Could you check a few things on this model? Use its own coordinates, in mm. Coordinates: 2 decimals unless noted, no trailing zeros. Write each loop counter-clockwise with the first axis right and the second up, starting at its lowest first coordinate (ties: lowest second). Pieces come first, ordered by that corner, then holes.
Autodesk Inventor part; units mm, degrees
ref_plane "РабПлоскость1" through (0, -6.05, 0) normal (1, 0, 0) x (0, 0, -1)
ref_plane "YZ Plane" through (0, 0, 0) normal (1, 0, 0) x (0, 1, 0)
ref_plane "XZ Plane" through (0, 0, 0) normal (0, 1, 0) x (-1, 0, 0)
sketch "Эскиз1" plane through (0, 0, 0) normal (0, 0, 1) x (1, 0, 0)
  circle A0 centre (0, 0) radius 4.05
  line L0 (-6.05, -6.05) -> (6.05, -6.05)
  line L1 (6.05, -6.05) -> (6.05, 6.05)
  line L2 (6.05, 6.05) -> (-6.05, 6.05)
  line L3 (-6.05, 6.05) -> (-6.05, -6.05)
  line L4 (-6.05, -6.05) -> (6.05, 6.05) construction
  line L5 (6.05, -6.05) -> (-6.05, 6.05) construction
  line L6 (0, 6.05) -> (0, 4.05)
  line L7 (-6.05, 0) -> (-4.05, 0)
  line L8 (-13, -3.05) -> (0, -3.05)
  line L9 (0, -3.05) -> (0, -6.05)
  line L10 (0, -6.05) -> (-13, -6.05)
  line L11 (-13, -6.05) -> (-13, -3.05)
  line L12 (13, -3.05) -> (0, -3.05)
  line L13 (0, -6.05) -> (13, -6.05)
  line L14 (13, -6.05) -> (13, -3.05)
  point P0 (0, -4.55)
  point P1 (0, -6.05)
  point P2 (2.6646, -3.05)
  point P3 (-2.6646, -3.05)
  dimension "d0" = 8.1
  dimension "d1" = 2
  dimension "d2" = 2
  dimension "d3" = 3
  dimension "d5" = 3
  dimension "d6" = 6.95
extrude "Выдавливание1" add sketch "Эскиз1" along normal blind 5.1 contours L12 L1 L0 L9 A0 | L9 L0 L3 L8 A0 | L12 L14 L13 L1 | L3 L10 L11 L8
sketch "Эскиз2" plane through (-13, -3.05, 0) normal (0, 1, 0) x (1, 0, 0)
  line L0 (0, 0) -> (0, -5.1)
  line L1 (0, -2.55) -> (2.4, -2.55)
  point P0 (13, 0)
  dimension "d9" = 2.4
ref_plane "РабПлоскость1" through (0, -6.05, 0) normal (1, 0, 0) x (0, 0, -1)
hole "Отверстие1" at (-10.6, -3.05, 2.55) direction (0, -1, 0) diameter 3.2 end through all
mirror "Зеркальное отражение1" about plane through (0, -6.05, 0) normal (1, 0, 0) of "Отверстие1"
fillet "Сопряжение1" radius 2.55 4 edges at (-13, -4.55, 5.1) (-13, -4.55, 0) (13, -4.55, 5.1) (13, -4.55, 0)
sketch "Эскиз3" plane through (-10.45, -6.05, 0) normal (0, -1, 0) x (1, 0, 0)
  arc A0 (20.9, 0) -> (20.9, 5.1) centre (20.9, 2.55) ccw
  line L0 (0, 5.1) -> (20.9, 5.1)
  arc A1 (0, 5.1) -> (0, 0) centre (0, 2.55) ccw
  line L1 (0, 0) -> (20.9, 0)
  circle A2 centre (-0.15, 2.55) radius 1.6
  circle A3 centre (21.05, 2.55) radius 1.6
  point P0 (10.45, 0)
extrude "Выдавливание2" add sketch "Эскиз3" along normal blind 7.05
properties part number "Стойка подшипника 3мм"
1. If we mould it in two halves opening along X, with no side actions, what happens to faces 1 (the face through (-12.273, -4.529, 4.333)), 2 (the face through (0.04, -4.05, 2.51)), 3 (the face through (0, -8, 0))? For each: pulls with the +X half, pulls with the -X half, needs draft (parallel to the pull), parting line crosses it, or undercut.
Verdict:
face 1: pulls with the -X half
face 2: undercut
face 3: needs draft
2. For pin 1 (1.3 mm diameter, centred on x = -11.5, z = 1.5, fed in from -Y); pin 2 (3 mm diameter, centred on x = -10.6, z = 2.55, fed in from +Y), each with a flat end and sliding along its axis, tell me the tip position at first contact or that it passes through.
Verdict:
pin 1: stops at y = -13.1
pin 2: passes through
3. Please list where these lines run through material, in increasing order: line 1 along X through (y, z) = (-4.75, 2.55); line 2 along Z through (x, y) = (10.6, -5.05); line 3 along X through (y, z) = (-11, 2.1).
Verdict:
line 1: x = -13 to -12.2, -9 to 9, 12.2 to 13
line 2: z = 0 to 0.95, 4.15 to 5.1
line 3: x = -12.96 to -12.14, -9.06 to 9.06, 12.14 to 12.96
4. I want a section at A-A on y = -5. Give the number of separate pieces and of enclosed holes in the cut face, plus the area to 3 significant figures.
Verdict:
separate pieces: 1
enclosed holes: 2
area: 111 mm2
5. I want a section at D-D on y = -11. Please give me the cut outline in (x, z), plus the area to 3 significant figures.
Verdict:
outline: (-10.45, 0) - (10.45, 0) arc R2.55 ccw to (10.45, 5.1) - (-10.45, 5.1) arc R2.55 ccw to start; hole circle Ø3.2 at (-10.6, 2.55); hole circle Ø3.2 at (10.6, 2.55)
area: 111 mm2
